from build123d import *

# Parameters (mm, degrees)
F0_W     = 21
F0_H     = 15
F1_DEPTH = 6
F3_DEPTH = 8
F4_R     = 2
F5_DEPTH = 3


with BuildPart() as f1:
    # F0 (on Top) → F1 (new body)
    with BuildSketch(Plane.XY):
        Rectangle(F0_W, F0_H)
    extrude(amount=F1_DEPTH)

    # F2 (on Right) → F3 (cut, symmetric)
    with BuildSketch(Plane.YZ):
        Polygon((5, 6), (-5, 6), (0, 2), align=None)
    extrude(amount=F3_DEPTH, both=True, mode=Mode.SUBTRACT)

    # F4 (on Top) → F5 (join)
    with BuildSketch(Plane.XY):
        with BuildLine():
            Line((-4, 12.5), (-4, 7.5))
            Line((-4, 7.5), (4, 7.5))
            Line((4, 7.5), (4, 12.5))
            ThreePointArc((4, 12.5), (0, 16.5), (-4, 12.5))
        make_face()
        with Locations((0, 12.5)):
            Circle(F4_R, mode=Mode.SUBTRACT)
        with BuildLine():
            Line((4, -7.5), (-4, -7.5))
            Line((-4, -7.5), (-4, -12.5))
            ThreePointArc((-4, -12.5), (0, -16.5), (4, -12.5))
            Line((4, -12.5), (4, -7.5))
        make_face()
        with Locations((0, -12.5)):
            Circle(F4_R, mode=Mode.SUBTRACT)
    extrude(amount=F5_DEPTH)


solid = f1.part
The listing builds one solid part. Answer for the finished solid, in the listing's coordinates (mm). A direction names the side the tool comes from. Round coordinates to 2 decimals unless told otherwise and drop trailing zeros. Write each loop counter-clockwise with the first axis right and the second up, starting at its lowest first coordinate (ties: lowest second). Pieces come first, ordered by that corner, then holes. Notation, with made-up numbers: M 78,44.5 L 136,44.5 A11 ccw 136,51.5 Z; hole C 50,-19.75 d1. An arc over 180 degrees is marked long. Write each question's results on one line, items separated by ' | '. Start each with the question number.
Item 1: Which of the six approach directions +Z, -Z, +X, -X, +Y, -Y give full straight-line access (tool end or side, diameter ignored) to faces 5 (the flat face through (0, -10, 3)), 6 (the flat face through (-4, 10, 1)), 7 (the flat face through (0.1, -2.5, 4)), 8 (the flat face through (0, 10, 3)), 9 (the flat face through (4, 10, 1))?
Item 2: Find section A-A on z = 5.2. Write down the section's boundary in (x, y).
Item 3: Find section B-B on x = 0. Write down the section's boundary in (y, z).
Item 4: Find section C-C on y = 13.5. Write down the section's boundary in (x, z), and give its area (3 significant figures).
Item 5: Given pin 1 Ø0.9 at (y, z) = (-9.5, 2) entering from +X; pin 2 Ø0.9 at (y, z) = (-9.5, 1) entering from -X; pin 3 Ø1.8 at (x, z) = (3, 3.5) entering from +Y, each flat-ended and moving along its own axis, determine where each tip first touches the part or whether it passes through.
Item 6: Straight lines are drawn through the part: probe 1 along Y at (x, z) = (0, 0.85); probe 2 along Y at (x, z) = (0, 2.35); probe 3 along Z at (x, y) = (3, 11.5). For each, find the intervals that lie inside material, in ascending order.
Item 7: Find section D-D on x = -5.75. Write down the section's boundary in (y, z), and give its area (3 significant figures).
Item 8: The mould has two halves that part along Y. Classify faces 1 (the cylindrical face through (0.1, 16.5, 1.5)), 2 (the cylindrical face through (-0.1, -16.5, 1.5)), 3 (the flat face through (10.5, 0, 3)), 4 (the flat face through (-8, 0, 4)): +Y half, -Y half, draft (parallel to the pull), parting line (faces both ways), or undercut.
Answer block:
1) face 5: +Z, +X, -X, -Y | face 6: +Z, -Z, -X, +Y | face 7: +Z | face 8: +Z, +X, -X, +Y | face 9: +Z, -Z, +X, +Y
2) outline: M -10.5,-7.5 L 10.5,-7.5 L 10.5,7.5 L -10.5,7.5 Z; hole M -8,-4 L 8,-4 L 8,4 L -8,4 Z
3) outline: M -16.5,0 L -14.5,0 L -14.5,3 L -16.5,3 Z; M -10.5,0 L 10.5,0 L 10.5,3 L 7.5,3 L 7.5,6 L 5,6 L 0,2 L -5,6 L -7.5,6 L -7.5,3 L -10.5,3 Z; M 14.5,0 L 16.5,0 L 16.5,3 L 14.5,3 Z
4) outline: M -3.87,0 L -1.73,0 L -1.73,3 L -3.87,3 Z; M 1.73,0 L 3.87,0 L 3.87,3 L 1.73,3 Z | area: 12.8 mm²
5) pin 1: stops at x = 4 | pin 2: stops at x = -4 | pin 3: stops at y = 15.81
6) probe 1: y = -16.5 to -14.5, -10.5 to 10.5, 14.5 to 16.5 | probe 2: y = -16.5 to -14.5, -10.5 to -0.44, 0.44 to 10.5, 14.5 to 16.5 | probe 3: z = 0 to 3
7) outline: M -7.5,0 L 7.5,0 L 7.5,6 L 5,6 L 0,2 L -5,6 L -7.5,6 Z | area: 70.0 mm²
8) face 1: +Y half | face 2: -Y half | face 3: draft | face 4: undercut
